The listing builds one solid part. Answer for the finished solid, in the listing's coordinates (mm). A direction names the side the tool comes from. Coordinates: 2 decimals unless noted, no trailing zeros. Order: outer loops, then holes, each group sorted by start corner. A loop starts at its lowest first (then second) coordinate and runs counter-clockwise, first axis right, second up. Notation, with made-up numbers: M -0.75,-16 L 57.25,-16 A32 cw 57.25,23 Z; hole C 85,-31 d5. An arc over 180 degrees is marked long. One line per item, written item: value. Start each with the question number.
Q1. Each of these flat-tipped pins is pushed along its axis until it touches: pin 1 Ø3.5 at (x, z) = (43.89, 35.27) entering from +Y; pin 2 Ø1.6 at (x, z) = (35.27, -43.89) entering from -Y. Where does it stop, or does it pass through?
Q2. Straight lines are drawn through the part: line 1 along Z through (x, y) = (30.5, 0.75); line 2 along Z through (x, y) = (-0.5, 0.8); line 3 along Z through (x, y) = (-12, 0.95). For each, find the intervals that lie inside material, in ascending order. Write a range as [from, to].
Q3. The part is cut by section A-A on z = 0. Give the vertices of the cut face in (x, y), then the cut area to 3 significant figures.
Q4. Determine the mould class of faces 4 (the cylindrical face through (-0.49, 0.689, 32.058)), 5 (the flat face through (-44.7, 0.69, -45.04)), 6 (the flat face through (-12, 1.397, 10)), 7 (the flat face through (44.75, 0.69, -44.99)) for opening direction X: pulls with the +X half, pulls with the -X half, needs draft (parallel to the pull), parting line crosses it, or undercut.
Q5. The part is cut by section D-D on z = 22.5. Give the vertices of the cut face in (x, y).
Q6. The part is cut by section C-C on y = 1. Give the number of separate pieces and of enclosed holes in the cut face, then the cut area to 3 significant figures.
Q7. The part is cut by section B-B on x = 0. Give the vertices of the cut face in (y, z).
Q8. For faces 1 (the cylindrical face through (46.52, 0.69, 39.04)), 2 (the cylindrical face through (38.86, 0.689, -46.664)), 3 (the cylindrical face through (38.8, 0.69, 46.71)), determine the directions among +Z, -Z, +X, -X, +Y, -Y from which every point of the face is accessible in a straight line to the end or side of a thin tool.
```python
from build123d import *

# Parameters (mm, degrees)
SKETCH1_R           = 1.015999988
SKETCH1_R_2         = 15
BOSS_EXTRUDE1_DEPTH = 1.397


with BuildPart() as part:
    # Sketch1 → Boss-Extrude1 (new body)
    with BuildSketch(Plane(origin=(0, 0, 0), x_dir=(1, 0, 0), z_dir=(0, 1, 0))):
        with BuildLine():
            Line((-44.657487237, -41.209177315), (-46.396043567, -42.947733627))
            ThreePointArc((-46.396043567, -42.947733627), (-46.470434262, -43.125880964), (-46.398093323, -43.304870453))
            Line((-46.398093323, -43.304870453), (-43.050556802, -46.730153525))
            ThreePointArc((-43.050556802, -46.730153525), (-42.865374815, -46.831022568), (-42.667823867, -46.757262447))
            Line((-42.667823867, -46.757262447), (-40.871772634, -44.961211232))
            ThreePointArc((-40.871772634, -44.961211232), (-38.831009245, -46.687575098), (-36.702263685, -48.30420423))
            ThreePointArc((-36.702263685, -48.30420423), (-33.138347002, -49.294565873), (-29.78114627, -47.741658512))
            ThreePointArc((-29.78114627, -47.741658512), (0, -32.054645119), (29.78114627, -47.741658512))
            ThreePointArc((29.78114627, -47.741658512), (33.138347002, -49.294565873), (36.702263685, -48.30420423))
            ThreePointArc((36.702263685, -48.30420423), (38.831009245, -46.687575098), (40.871772634, -44.961211232))
            Line((40.871772634, -44.961211232), (42.667823867, -46.757262447))
            ThreePointArc((42.667823867, -46.757262447), (42.865374815, -46.831022568), (43.050556802, -46.730153525))
            Line((43.050556802, -46.730153525), (46.398093323, -43.304870453))
            ThreePointArc((46.398093323, -43.304870453), (46.470434262, -43.125880964), (46.396043567, -42.947733627))
            Line((46.396043567, -42.947733627), (44.657487237, -41.209177315))
            ThreePointArc((44.657487237, -41.209177315), (46.545191357, -39.007785017), (48.30420423, -36.702263685))
            ThreePointArc((48.30420423, -36.702263685), (49.294565905, -33.13834702), (47.741658512, -29.78114627))
            ThreePointArc((47.741658512, -29.78114627), (41.575395348, 0), (47.741658512, 29.78114627))
            ThreePointArc((47.741658512, 29.78114627), (49.294565905, 33.13834702), (48.30420423, 36.702263685))
            ThreePointArc((48.30420423, 36.702263685), (46.545191357, 39.007785017), (44.657487237, 41.209177315))
            Line((44.657487237, 41.209177315), (46.396043567, 42.947733627))
            ThreePointArc((46.396043567, 42.947733627), (46.470434262, 43.125880964), (46.398093323, 43.304870453))
            Line((46.398093323, 43.304870453), (43.050556802, 46.730153525))
            ThreePointArc((43.050556802, 46.730153525), (42.865374815, 46.831022568), (42.667823867, 46.757262447))
            Line((42.667823867, 46.757262447), (40.871772634, 44.961211232))
            ThreePointArc((40.871772634, 44.961211232), (38.831009245, 46.687575098), (36.702263685, 48.30420423))
            ThreePointArc((36.702263685, 48.30420423), (33.138347002, 49.294565873), (29.78114627, 47.741658512))
            ThreePointArc((29.78114627, 47.741658512), (0, 32.054645119), (-29.78114627, 47.741658512))
            ThreePointArc((-29.78114627, 47.741658512), (-33.138347002, 49.294565873), (-36.702263685, 48.30420423))
            ThreePointArc((-36.702263685, 48.30420423), (-38.831009245, 46.687575098), (-40.871772634, 44.961211232))
            Line((-40.871772634, 44.961211232), (-42.667823867, 46.757262447))
            ThreePointArc((-42.667823867, 46.757262447), (-42.865374815, 46.831022568), (-43.050556802, 46.730153525))
            Line((-43.050556802, 46.730153525), (-46.398093323, 43.304870453))
            ThreePointArc((-46.398093323, 43.304870453), (-46.470434262, 43.125880964), (-46.396043567, 42.947733627))
            Line((-46.396043567, 42.947733627), (-44.657487237, 41.209177315))
            ThreePointArc((-44.657487237, 41.209177315), (-46.545191357, 39.007785017), (-48.30420423, 36.702263685))
            ThreePointArc((-48.30420423, 36.702263685), (-49.294565905, 33.13834702), (-47.741658512, 29.78114627))
            ThreePointArc((-47.741658512, 29.78114627), (-41.575395348, 0), (-47.741658512, -29.78114627))
            ThreePointArc((-47.741658512, -29.78114627), (-49.294565905, -33.13834702), (-48.30420423, -36.702263685))
            ThreePointArc((-48.30420423, -36.702263685), (-46.545191357, -39.007785017), (-44.657487237, -41.209177315))
        make_face()
        with Locations(Location((-35.273880272, -43.89492624, 0), (0, 0, 90))):
            Circle(SKETCH1_R, mode=Mode.SUBTRACT)
        with Locations(Location((-43.894926149, -35.273880364, 0), (0, 0, 270))):
            Circle(SKETCH1_R, mode=Mode.SUBTRACT)
        with Locations(Location((-31.299173944, -31.299174035, 0), (0, 0, 270))):
            Circle(SKETCH1_R, mode=Mode.SUBTRACT)
        with Locations(Location((43.894926149, -35.273880364, 0), (0, 0, 90))):
            Circle(SKETCH1_R, mode=Mode.SUBTRACT)
        with Locations(Location((35.273880272, -43.89492624, 0), (0, 0, 270))):
            Circle(SKETCH1_R, mode=Mode.SUBTRACT)
        with Locations(Location((31.299173944, -31.299174035, 0), (0, 0, 90))):
            Circle(SKETCH1_R, mode=Mode.SUBTRACT)
        with Locations(Location((-35.273880272, 43.89492624, 0), (0, 0, 270))):
            Circle(SKETCH1_R, mode=Mode.SUBTRACT)
        with Locations(Location((-31.299173944, 31.299174035, 0), (0, 0, 90))):
            Circle(SKETCH1_R, mode=Mode.SUBTRACT)
        with Locations(Location((-43.894926149, 35.273880364, 0), (0, 0, 90))):
            Circle(SKETCH1_R, mode=Mode.SUBTRACT)
        with Locations(Location((43.894926149, 35.273880364, 0), (0, 0, 270))):
            Circle(SKETCH1_R, mode=Mode.SUBTRACT)
        with Locations(Location((35.273880272, 43.89492624, 0), (0, 0, 90))):
            Circle(SKETCH1_R, mode=Mode.SUBTRACT)
        with Locations(Location((31.299173944, 31.299174035, 0), (0, 0, 270))):
            Circle(SKETCH1_R, mode=Mode.SUBTRACT)
        with Locations(Location((0, 0, 0), (0, 0, 270))):
            Circle(SKETCH1_R_2, mode=Mode.SUBTRACT)
    extrude(amount=BOSS_EXTRUDE1_DEPTH)


solid = part.part
```
Output:
1. pin 1: stops at y = 1.4
1. pin 2: passes through
2. line 1: z = [-48.34, -31.93], [-30.67, 30.67], [31.93, 48.34]
2. line 2: z = [-32.06, -14.99], [14.99, 32.06]
2. line 3: z = [-34.11, -9], [9, 34.11]
3. outline: M -41.58,0 L -15,0 L -15,1.4 L -41.58,1.4 Z; M 15,0 L 41.58,0 L 41.58,1.4 L 15,1.4 Z
3. area: 74.3 mm^2
4. face 4: undercut
4. face 5: pulls with the -X half
4. face 6: needs draft
4. face 7: pulls with the +X half
5. outline: M -45.03,0 L 45.03,0 L 45.03,1.4 L -45.03,1.4 Z
6. separate pieces: 1
6. enclosed holes: 13
6. area: 6,500 mm^2
7. outline: M 0,-32.05 L 1.4,-32.05 L 1.4,-15 L 0,-15 Z; M 0,15 L 1.4,15 L 1.4,32.05 L 0,32.05 Z
8. face 1: +X, +Y, -Y
8. face 2: -Z, +Y, -Y
8. face 3: +Z, +Y, -Y
